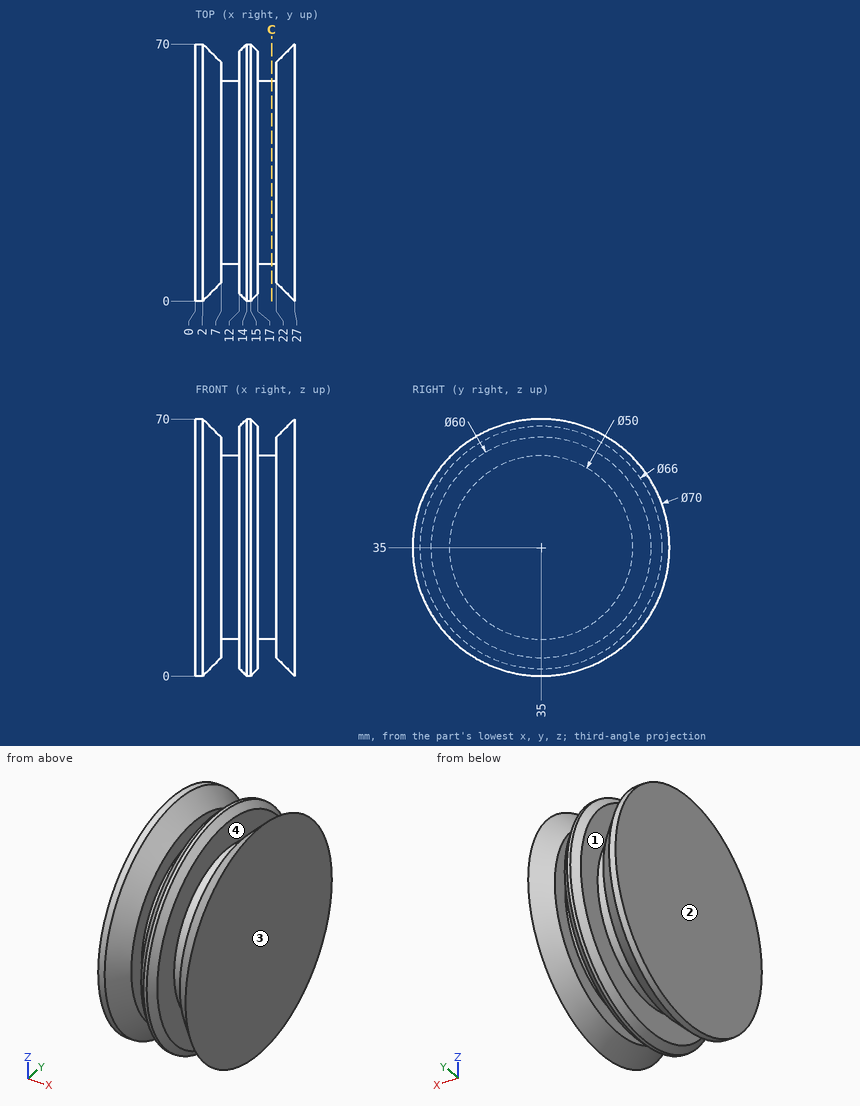
Geometry: see drawing. Coordinates: mm, zero at the bounding-box minimum. Round coordinates to 2 decimals unless told otherwise and drop trailing zeros. Loops run counter-clockwise (first coordinate to the right, second up) from the corner with the lowest first, then second, coordinate; pieces in that order, holes last. Notation, with made-up numbers: (23.25, 13) - (30.25, 13) arc R20 cw to (30.25, 20) - close; hole circle Ø11 at (-5.75, -4.5). An arc over 180 degrees is marked (long way). One line per item, written item: value. Start each with the question number.
(1) Draft query along X for the marked faces 1, 2, 3 and 4. Return one class per face: +X half, -X half, draft (parallel to the pull), parting line (faces both ways), or undercut.
(2) Section C-C, the plane x = 20.75. Return loops of the section in (y, z).
(3) Contact query for flat-ended pins moving along their axis: P1, Ø5, axis at x = 24, y = 42.5, coming from the -Z side; P2, Ø6, axis at y = 50, z = 27, coming from the -X side; P3, Ø4, axis at x = 3, y = 10, coming from the -Z side; P4, Ø8, axis at x = 9, z = 26, coming from the +Y side. Output: stop coordinate, or through.
(4) Ray query, line 1 (X direction, y = 42, z = 10); line 2 (X direction, y = 51.5, z = 9); line 3 (Z direction, x = 14.25, y = 10.5) (3 decimals). Return the intervals inside material, ascending. Write a range as [from, to].
Results below:
1. face 1: undercut
1. face 2: -X half
1. face 3: +X half
1. face 4: undercut
2. outline: circle Ø50 at (35, 35)
3. P1: z = 1.27
3. P2: x = 0
3. P3: z = 8.85
3. P4: y = 67.92
4. line 1: [0, 7], [12, 17], [22, 27]
4. line 2: [0, 6.21], [12, 17], [22.79, 27]
4. line 3: [10.005, 59.995]
